For this review, take the finished solid that the model builds, in its own axes (mm). A direction names the side the tool comes from. Round coordinates to 2 decimals unless told otherwise and drop trailing zeros. Write each loop counter-clockwise with the first axis right and the second up, starting at its lowest first coordinate (ties: lowest second). Pieces come first, ordered by that corner, then holes. Notation, with made-up numbers: (-27.5, 9) -> (4.5, 9) arc R26 ccw to (4.5, 28) -> close; hole circle Ø2 at (14, 84). An arc over 180 degrees is marked (long way). Answer in a Markdown table with one row per item.
Autodesk Inventor part; units mm, degrees
ref_plane "YZ Plane" through (0, 0, 0) normal (1, 0, 0) x (0, 1, 0)
ref_plane "XZ Plane" through (0, 0, 0) normal (0, 1, 0) x (-1, 0, 0)
ref_plane "XY Plane" through (0, 0, 0) normal (0, 0, 1) x (1, 0, 0)
sketch "Sketch1" plane through (0, 0, 0) normal (0, 0, 1) x (1, 0, 0)
  line L0 (7.3323, 0) -> (3.6662, -6.35)
  line L1 (3.6662, -6.35) -> (-3.6662, -6.35)
  line L2 (-3.6662, -6.35) -> (-7.3323, 0)
  line L3 (-7.3323, 0) -> (-3.6662, 6.35)
  line L4 (-3.6662, 6.35) -> (3.6662, 6.35)
  line L5 (3.6662, 6.35) -> (7.3323, 0)
  point P0 (0, 0)
  point P1 (0, 0)
  dimension "d0" = 12.7
extrude "Extrusion1" add sketch "Sketch1" along normal mid plane 343.535
sketch "Sketch2" plane through (0, 0, 171.7675) normal (0, 0, 1) x (1, 0, 0)
  circle A0 centre (0, 0) radius 5.9436
  dimension "d3" = 11.8872
extrude "Extrusion2" add sketch "Sketch2" along normal blind 0.9906
sketch "Sketch3" plane through (0, 0, 172.7581) normal (0, 0, 1) x (1, 0, 0)
  circle A0 centre (0, 0) radius 5.9436
  line L0 (3.6662, -6.35) -> (7.3323, 0)
  line L1 (7.3323, 0) -> (3.6662, 6.35)
  line L2 (3.6662, 6.35) -> (-3.6662, 6.35)
  line L3 (-3.6662, 6.35) -> (-7.3323, 0)
  line L4 (-7.3323, 0) -> (-3.6662, -6.35)
  line L5 (-3.6662, -6.35) -> (3.6662, -6.35)
  circle A1 centre (0, 0) radius 6.35
extrude "Extrusion3" add sketch "Sketch3" along normal blind 1.5875 contours A0 | A1
mirror "Mirror1" about plane through (0, 0, 0) normal (0, 0, 1) of "Extrusion2", "Extrusion3"
sketch "Sketch4" plane through (-3.6662, -6.35, -171.7675) normal (-0.866, -0.5, 0) x (0, 0, 1)
  line L0 (61.571, -23.211) -> (381.4095, -23.211)
  line L1 (381.4095, -23.211) -> (381.4095, 34.5749)
  line L2 (381.4095, 34.5749) -> (61.571, 34.5749)
  line L3 (61.571, 34.5749) -> (61.571, -23.211)
  point P0 (171.7675, 3.6662)
extrude "Extrusion4" cut sketch "Sketch4" against normal blind 25.4
sketch "Sketch5" plane through (-3.6662, -6.35, -110.1965) normal (0, 0, 1) x (1, 0, 0)
  circle A0 centre (3.6662, 6.35) radius 6.35
  dimension "d10" = 12.7
extrude "Extrusion5" add sketch "Sketch5" along normal blind 6.35
properties part number "ARM_010_2.75inHexShaft" material "Aluminum 6061"
1) Consider section C-C on y = 5. State the section outline as (x, z) points, then the cut area to 3 significant figures.
Solved:
| item | result |
|---|---|
| outline | (-4.45, -171.77) -> (-3.21, -171.77) -> (-3.21, -172.76) -> (-3.91, -172.76) -> (-3.91, -174.35) -> (3.91, -174.35) -> (3.91, -172.76) -> (3.21, -172.76) -> (3.21, -171.77) -> (4.45, -171.77) -> (4.45, -110.2) -> (3.91, -110.2) -> (3.91, -103.85) -> (-3.91, -103.85) -> (-3.91, -110.2) -> (-4.45, -110.2) -> close |
| area | 616 mm² |
2) Mouldability with a two-part tool opening along Z and no side actions: class faces 1 (the flat face through (5.474, 3.219, -141.413)), 2 (the cylindrical face through (5.669, 1.785, -172.256)), 3 (the flat face through (-3, -6, -110.196)) as pulls with the +Z half, pulls with the -Z half, needs draft (parallel to the pull), parting line crosses it, or undercut.
Solved:
| item | result |
|---|---|
| face 1 | needs draft |
| face 2 | undercut |
| face 3 | pulls with the +Z half |
3) For faces 4 (the flat face through (3, -6, -110.196)), 5 (the flat face through (-7, 0, -110.196)), 6 (the flat face through (3, 6, -110.196)), 7 (the cylindrical face through (-1.38, -6.2, -173.54)), 8 (the flat face through (-3, 6, -110.196)), list the 3-axis set-ups (+Z, -Z, +X, -X, +Y, -Y) from which the entire face can be reached by the end or side of a thin tool; tool diameter is ignored.
Solved:
| item | result |
|---|---|
| face 4 | +Z, +X, -Y |
| face 5 | +Z, -X |
| face 6 | +Z, +X, +Y |
| face 7 | -Z |
| face 8 | +Z, -X, +Y |
4) For line 1 (Z direction, x = 1.5, y = 6.25); line 2 (X direction, y = 4, z = -156); line 3 (Y direction, x = 6.75, z = -163), list the stretches that pass through material, from the lowest coordinate up. Write a range as [from, to].
Solved:
| item | result |
|---|---|
| line 1 | [-171.77, -110.2] |
| line 2 | [-5.02, 5.02] |
| line 3 | [-1.01, 1.01] |
5) Consider section B-B on y = -2.5. State the section outline as (x, z) points.
Solved:
| item | result |
|---|---|
| outline | (-5.89, -171.77) -> (-5.39, -171.77) -> (-5.39, -172.76) -> (-5.84, -172.76) -> (-5.84, -174.35) -> (5.84, -174.35) -> (5.84, -172.76) -> (5.39, -172.76) -> (5.39, -171.77) -> (5.89, -171.77) -> (5.89, -110.2) -> (5.84, -110.2) -> (5.84, -103.85) -> (-5.84, -103.85) -> (-5.84, -110.2) -> (-5.89, -110.2) -> close |
6) Clearance check with flat-ended pins moving along their axes: pin 1 Ø4 at (y, z) = (-2.5, -139.5) entering from +X; pin 2 Ø1.6 at (x, y) = (3.5, 5.5) entering from +Z; pin 3 Ø0.5 at (x, y) = (6.5, 1.5) entering from +Z; pin 4 Ø1 at (x, z) = (-4.5, -125) entering from -Y. State where each tip first meets the part, or that it passes through.
Solved:
| item | result |
|---|---|
| pin 1 | x = 7.04 |
| pin 2 | z = -103.85 |
| pin 3 | z = -110.2 |
| pin 4 | y = -5.77 |
7) Consider section A-A on z = -137.5. State the section outline as (x, y) points, then the cut area to 3 significant figures.
Solved:
| item | result |
|---|---|
| outline | (-7.33, 0) -> (-3.67, -6.35) -> (3.67, -6.35) -> (7.33, 0) -> (3.67, 6.35) -> (-3.67, 6.35) -> close |
| area | 140 mm² |
